```python
from build123d import *

# Parameters (mm, degrees)
F0_W     = 406.4
F0_H     = 660.4
F1_DEPTH = 6.35
F2_W     = 152.4
F2_H     = 241.3
F3_DEPTH = 6.351
F4_R     = 3.175
F5_DEPTH = 12.7


with BuildPart() as f1:
    # F0 (on Front) → F1 (new body)
    with BuildSketch(Plane.XZ):
        with Locations((203.2, 330.2)):
            Rectangle(F0_W, F0_H)
    extrude(amount=F1_DEPTH)

    # F2 (on face) → F3 (cut, through all)
    with BuildSketch(Plane.XZ.offset(6.35)):
        with Locations((114.3, 482.6)):
            Rectangle(F2_W, F2_H)
        with Locations((298.45, 482.6)):
            Rectangle(F2_W, F2_H)
    extrude(amount=-F3_DEPTH, mode=Mode.SUBTRACT)

    # F4 (on face) → F5 (join)
    with BuildSketch(Plane.XZ.offset(6.35)):
        with Locations((44.45, 615.95)):
            Circle(F4_R)
        with Locations((184.15, 615.95)):
            Circle(F4_R)
        with Locations((44.45, 349.25)):
            Circle(F4_R)
        with Locations((184.15, 349.25)):
            Circle(F4_R)
        with Locations((228.6, 615.95)):
            Circle(F4_R)
        with Locations((368.3, 615.95)):
            Circle(F4_R)
        with Locations((228.6, 349.25)):
            Circle(F4_R)
        with Locations((368.3, 349.25)):
            Circle(F4_R)
    extrude(amount=F5_DEPTH)


solid = f1.part
```
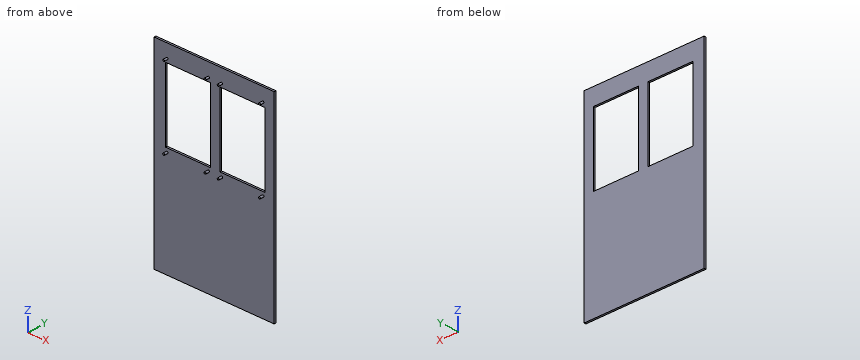
Model file for the job. Use its own axes, mm. Give positions to 0.01 mm unless a question says otherwise; leave off trailing zeros. Write each loop counter-clockwise with the first axis right and the second up, starting at its lowest first coordinate (ties: lowest second). Pieces come first, ordered by that corner, then holes. Notation, with made-up numbers: (20, 62) - (77, 62) arc R12 cw to (77, 67) - close; hole circle Ø3 at (17, -39.5). An arc over 180 degrees is marked (long way). One line per question, with ' | ' between items. Start each with the question number.
(1) Slice it at D-D on x = 207.5. Write the cut outline in (y, z).
(2) Wall check: line 1 along X through (y, z) = (-4.25, 367); line 2 along Z through (x, y) = (186.5, -3.75); line 3 along Y through (x, z) = (380.5, 493). Give the ranges that are in metal, low to high. Write a range as from..to.
(3) Pin check, flat tip, straight feed: P1, Ø3, axis at x = 303, y = -6, coming from the -Z side. Stop position of the tip, or through.
(4) Slice it at A-A on x = 108.5. Write the cut outline in (y, z), plus the area to 3 significant figures.
(5) Slice it at C-C on z = 471.5. Write the cut outline in (x, y).
(6) Slice it at B-B on y = -12. Write the cut outline in (x, z) (3 decimals).
Results below:
1) outline: (-6.35, 0) - (0, 0) - (0, 660.4) - (-6.35, 660.4) - close
2) line 1: 0..38.1, 190.5..222.25, 374.65..406.4 | line 2: 0..361.95, 603.25..660.4 | line 3: -6.35..0
3) P1: z = 0
4) outline: (-6.35, 0) - (0, 0) - (0, 361.95) - (-6.35, 361.95) - close; (-6.35, 603.25) - (0, 603.25) - (0, 660.4) - (-6.35, 660.4) - close | area: 2,660 mm^2
5) outline: (0, -6.35) - (38.1, -6.35) - (38.1, 0) - (0, 0) - close; (190.5, -6.35) - (222.25, -6.35) - (222.25, 0) - (190.5, 0) - close; (374.65, -6.35) - (406.4, -6.35) - (406.4, 0) - (374.65, 0) - close
6) outline: circle Ø6.35 at (44.45, 349.25); circle Ø6.35 at (44.45, 615.95); circle Ø6.35 at (184.15, 349.25); circle Ø6.35 at (184.15, 615.95); circle Ø6.35 at (228.6, 349.25); circle Ø6.35 at (228.6, 615.95); circle Ø6.35 at (368.3, 349.25); circle Ø6.35 at (368.3, 615.95)
